The listing builds one solid part. Answer for the finished solid, in the listing's coordinates (mm). A direction names the side the tool comes from. Coordinates: 2 decimals unless noted, no trailing zeros. Order: outer loops, then holes, each group sorted by start corner. A loop starts at its lowest first (then second) coordinate and runs counter-clockwise, first axis right, second up.
from build123d import *

# Parameters (mm, degrees)
SKETCH1_R               = 3.649213309
BOSS_EXTRUDE1_DEPTH     = 2.54
SKETCH1_R_2             = 4.666904756
SKETCH1_R_3             = 2.193652513
BOSS_EXTRUDE1_2_DEPTH   = 2.54
BOSS_EXTRUDE1_3_DEPTH   = 2.54
BOSS_EXTRUDE1_4_DEPTH   = 2.54
SKETCH2_R               = 2.193652513
SKETCH2_R_2             = 2.221197288
SKETCH2_R_3             = 3.649213309
BOSS_EXTRUDE2_DEPTH     = 2.54
SKETCH4_R               = 2.193652513
BOSS_EXTRUDE3_DEPTH     = 2.54
BOSS_EXTRUDE4_REACH     = 60.675
SKETCH5_W               = 19.155946822
SKETCH5_H               = 5.08
SKETCH6_W               = 19.155946822
SKETCH6_H               = 5.30085264
BOSS_EXTRUDE5_DEPTH     = 6.35
SKETCH7_W               = 19.155946822
SKETCH7_H               = 3.58914736
SKETCH7_H_2             = 5.30085264
BOSS_EXTRUDE6_DEPTH     = 6.349999999
CUT_EXTRUDE1_DEPTH      = 113.695579137
BOSS_EXTRUDE7_DEPTH     = 2.54
CUT_EXTRUDE2_DEPTH      = 107.988040918
CUT_EXTRUDE2_DEPTH_BACK = 107.988040918


with BuildPart() as part:
    # Sketch1 → Boss-Extrude1 (new body)
    with BuildSketch(Plane.XY):
        with Locations((-8.202026589, 4.509084108)):
            Circle(SKETCH1_R)
    extrude(amount=BOSS_EXTRUDE1_DEPTH)



with BuildPart() as body_2:
    # Sketch1 → Boss-Extrude1 2 (new body)
    with BuildSketch(Plane.XY):
        with Locations((-3.3, 41.15)):
            Circle(SKETCH1_R_2)
        with Locations((-3.3, 41.15)):
            Circle(SKETCH1_R_3, mode=Mode.SUBTRACT)
    extrude(amount=BOSS_EXTRUDE1_2_DEPTH)


with BuildPart() as body_3:
    # Sketch1 → Boss-Extrude1 3 (new body)
    with BuildSketch(Plane.XY):
        with Locations((-32.26, 41.15)):
            Circle(SKETCH1_R_2)
        with Locations((-32.26, 41.15)):
            Circle(SKETCH1_R_3, mode=Mode.SUBTRACT)
    extrude(amount=BOSS_EXTRUDE1_3_DEPTH)


with BuildPart() as body_4:
    # Sketch1 → Boss-Extrude1 4 (new body)
    with BuildSketch(Plane.XY):
        with Locations((-27.357973411, 4.509084108)):
            Circle(SKETCH1_R)
    extrude(amount=BOSS_EXTRUDE1_4_DEPTH)


with BuildPart() as part_1:
    add(part.part)

    add(body_2.part)  # Boss-Extrude2 merges body 2

    add(body_3.part)  # Boss-Extrude2 merges body 3

    add(body_4.part)  # Boss-Extrude2 merges body 4
    # Sketch2 → Boss-Extrude2 (add)
    # profile 1 of 5: a face of its own
    with BuildSketch(Plane.XY.offset(2.54)):
        with BuildLine():
            ThreePointArc((-8.202026589, 0.859870799), (-10.782410066, 7.089467585), (-4.552813279, 4.509084108))
            Line((-4.552813279, 4.509084108), (1.129473488, 39.680386235))
            ThreePointArc((1.129473488, 39.680386235), (-7.084081624, 38.418566994), (-3.3, 45.816904756))
            Line((-3.3, 45.816904756), (-32.26, 45.816904756))
            ThreePointArc((-32.26, 45.816904756), (-28.96, 44.45), (-27.593095244, 41.15))
            ThreePointArc((-27.593095244, 41.15), (-31.515665024, 36.542835423), (-36.689473488, 39.680386235))
            Line((-36.689473488, 39.680386235), (-31.007186721, 4.509084108))
            ThreePointArc((-31.007186721, 4.509084108), (-27.357973411, 8.158297418), (-23.708760102, 4.509084108))
            ThreePointArc((-23.708760102, 4.509084108), (-24.777589934, 1.928700631), (-27.357973411, 0.859870799))
            Line((-27.357973411, 0.859870799), (-8.202026589, 0.859870799))
        make_face()
    # profile 2 of 5: a face of its own
    with BuildSketch(Plane.XY.offset(2.54)):
        with BuildLine():
            ThreePointArc((-3.3, 45.816904756), (-7.084081624, 38.418566994), (1.129473488, 39.680386235))
            Line((1.129473488, 39.680386235), (1.366904756, 41.15))
            ThreePointArc((1.366904756, 41.15), (0, 44.45), (-3.3, 45.816904756))
        make_face()
        with Locations((-3.3, 41.15)):
            Circle(SKETCH2_R, mode=Mode.SUBTRACT)
    # profile 3 of 5: a face of its own
    with BuildSketch(Plane.XY.offset(2.54)):
        with BuildLine():
            ThreePointArc((-27.593095244, 41.15), (-28.96, 44.45), (-32.26, 45.816904756))
            ThreePointArc((-32.26, 45.816904756), (-35.56, 44.45), (-36.926904756, 41.15))
            Line((-36.926904756, 41.15), (-36.689473488, 39.680386235))
            ThreePointArc((-36.689473488, 39.680386235), (-31.515665024, 36.542835423), (-27.593095244, 41.15))
        make_face()
        with Locations((-32.26, 41.15)):
            Circle(SKETCH2_R_2, mode=Mode.SUBTRACT)
    # profile 4 of 5: a face of its own
    with BuildSketch(Plane.XY.offset(2.54)):
        with Locations(Location((-27.357973411, 4.509084108, 0), (0, 0, 180))):
            Circle(SKETCH2_R_3)
    # profile 5 of 5: a face of its own
    with BuildSketch(Plane.XY.offset(2.54)):
        with Locations((-8.202026589, 4.509084108)):
            Circle(SKETCH2_R_3)
    extrude(amount=BOSS_EXTRUDE2_DEPTH)

    # Sketch4 → Boss-Extrude3 (add)
    with BuildSketch(Plane.XY.offset(5.08)):
        with BuildLine():
            Line((-4.552813279, 4.509084108), (1.366904756, 41.15))
            ThreePointArc((1.366904756, 41.15), (0, 44.45), (-3.3, 45.816904756))
            Line((-3.3, 45.816904756), (-32.26, 45.816904756))
            ThreePointArc((-32.26, 45.816904756), (-35.56, 44.45), (-36.926904756, 41.15))
            Line((-36.926904756, 41.15), (-31.007186721, 4.509084108))
            ThreePointArc((-31.007186721, 4.509084108), (-29.938356889, 1.928700631), (-27.357973411, 0.859870799))
            Line((-27.357973411, 0.859870799), (-8.202026589, 0.859870799))
            ThreePointArc((-8.202026589, 0.859870799), (-5.621643111, 1.928700631), (-4.552813279, 4.509084108))
        make_face()
        with Locations((-3.3, 41.15)):
            Circle(SKETCH4_R, mode=Mode.SUBTRACT)
        with Locations((-32.26, 41.15)):
            Circle(SKETCH4_R, mode=Mode.SUBTRACT)
    extrude(amount=BOSS_EXTRUDE3_DEPTH)

    # Boss-Extrude4: up to this plane
    boss_extrude4_end = Plane(origin=(-92.143596389, -1.511792321, -30.321031804), z_dir=(0, 0.9583363932007225, 0.2856420092826512))
    # Sketch5 → Boss-Extrude4 (add, up to the surface)
    with BuildSketch(Plane.XZ.offset(-0.859870799), mode=Mode.PRIVATE) as boss_extrude4_sk1:
        with Locations((-17.78, 5.08)):
            Rectangle(SKETCH5_W, SKETCH5_H)
    boss_extrude4_tool1 = split(extrude(boss_extrude4_sk1.sketch, amount=BOSS_EXTRUDE4_REACH, mode=Mode.PRIVATE), bisect_by=boss_extrude4_end, keep=Keep.BOTH, mode=Mode.PRIVATE)
    add(boss_extrude4_tool1.solids().sort_by_distance((-17.78, 0.859871, 5.08))[0])

    # Sketch6 → Boss-Extrude5 (add)
    with BuildSketch(Plane(origin=(0, -9.68855673, -2.887773887), x_dir=(1, 0, 0), z_dir=(0, -0.9583363932007226, -0.2856420092826512))):
        with Locations((-17.78, 8.314172293)):
            Rectangle(SKETCH6_W, SKETCH6_H)
    extrude(amount=BOSS_EXTRUDE5_DEPTH)

    # Sketch7 → Boss-Extrude6 (add)
    with BuildSketch(Plane(origin=(0, -15.773992827, -4.701600646), x_dir=(1, 0, 0), z_dir=(0, -0.9583363932007226, -0.2856420092826512))):
        Polygon((-90.857973411, 5.663745973), (-27.357973411, 5.663745973), (-27.357973411, 10.964598613), (-27.357973411, 14.553745973), (-90.857973411, 14.553745973), align=None)
        with Locations((-17.78, 12.759172293)):
            Rectangle(SKETCH7_W, SKETCH7_H)
        with Locations((-17.78, 8.314172293)):
            Rectangle(SKETCH7_W, SKETCH7_H_2)
        Polygon((-8.202026589, 10.964598613), (-8.202026589, 5.663745973), (55.297973411, 5.663745973), (55.297973411, 14.553745973), (-8.202026589, 14.553745973), align=None)
    extrude(amount=-BOSS_EXTRUDE6_DEPTH)

    # Sketch9 → Cut-Extrude1 (cut, through all)
    with BuildSketch(Plane(origin=(0, 45.816904756, 0), x_dir=(1, 0, 0), z_dir=(0, 1, 0))):
        Polygon((-3.3, -7.62), (-17.78, -7.62), (-17.78, -45.955901378), (77.021856541, -45.955901378), (77.021856541, -7.62), align=None)
        Polygon((-17.78, -45.955901378), (-17.78, -7.62), (-32.26, -7.62), (-120.520571542, -7.62), (-120.520571542, -45.955901378), align=None)
    extrude(amount=-CUT_EXTRUDE1_DEPTH, mode=Mode.SUBTRACT)

    # Sketch10 → Boss-Extrude7 (add)
    with BuildSketch(Plane(origin=(0, -1.61780378, 5.427773887), x_dir=(-1, 0, 0), z_dir=(0, 0.28564200928265115, -0.9583363932007226))):
        Polygon((27.357973411, -10.109766049), (8.202026589, -10.109766049), (-55.297973411, -10.109766049), (-55.297973411, -16.459766048), (90.857973411, -16.459766048), (90.857973411, -10.109766049), align=None)
    extrude(amount=BOSS_EXTRUDE7_DEPTH)

    # Sketch11 → Cut-Extrude2 (cut, two sides: drawn at the far end of the back side and taken through both)
    with BuildSketch(Plane(origin=(0, -9.688556731, -2.887773887), x_dir=(1, 0, 0), z_dir=(0, 0.9583363932007284, 0.28564200928263184)).offset(-CUT_EXTRUDE2_DEPTH_BACK)):
        with BuildLine():
            Line((-41.109605197, -5.294172293), (-83.237973411, -5.294172293))
            ThreePointArc((-83.237973411, -5.294172293), (-84.475410278, -5.806735425), (-84.987973411, -7.044172293))
            ThreePointArc((-84.987973411, -7.044172293), (-84.475410278, -8.28160916), (-83.237973411, -8.794172293))
            Line((-83.237973411, -8.794172293), (-41.109605197, -8.794172293))
            ThreePointArc((-41.109605197, -8.794172293), (-39.359605197, -7.044172293), (-41.109605197, -5.294172293))
        make_face()
        with BuildLine():
            Line((5.549605197, -8.794172293), (47.677973411, -8.794172293))
            ThreePointArc((47.677973411, -8.794172293), (49.427973411, -7.044172293), (47.677973411, -5.294172293))
            Line((47.677973411, -5.294172293), (5.549605197, -5.294172293))
            ThreePointArc((5.549605197, -5.294172293), (3.799605197, -7.044172293), (5.549605197, -8.794172293))
        make_face()
    extrude(amount=CUT_EXTRUDE2_DEPTH + CUT_EXTRUDE2_DEPTH_BACK, mode=Mode.SUBTRACT)


solid = part_1.part
(1) The mould has two halves that part along X. Classify faces 6 (the flat face through (-27, 5, 0)), 7 (the flat face through (-8.202, -5, 5)), 8 (the flat face through (26.909, -14.286, 1.266)): pulls with the +X half, pulls with the -X half, needs draft (parallel to the pull), parting line crosses it, or undercut.
(2) Find the intervals of material crossed by probe 1 along Y at (x, z) = (-32.26, 1.55); probe 2 along Z at (x, y) = (-14, 43); probe 3 along Y at (x, z) = (-37, 6), in increasing order.
(3) Find section B-B on y = 16. Determine the outline of the cut face in (x, z).
(4) Find section C-C on x = -26. Determine the outline of the cut face in (y, z), then the cut area to 3 significant figures.
(5) Given pin 1 Ø2 at (x, z) = (-73, -0.5) entering from +Y; pin 2 Ø7.5 at (x, y) = (-3.5, 42.5) entering from -Z; pin 3 Ø2.5 at (x, y) = (-32.26, 41.15) entering from +Z; pin 4 Ø4 at (x, z) = (0.5, 0.5) entering from +Y, each flat-ended and moving along its own axis, determine where each tip first touches the part or whether it passes through.
(6) Find section D-D on x = -10. Determine the outline of the cut face in (y, z).
(7) A tool of negligible diameter and unlimited length cuts with its end or side. For faces 1 (the cylindrical face through (-35.7, 44.304, 2.91)), 2 (the cylindrical face through (49.428, -14.797, 2.98)), 3 (the flat face through (-62.47, -15.29, 4.62)), 4 (the flat face through (-1, 40, 0)), 5 (the flat face through (-61.879, -14.286, 1.266)), from which of +Z, -Z, +X, -X, +Y, -Y can it reach the whole face along a straight path? Write none if from no direction.
(8) Find section A-A on x = -73. Determine the outline of the cut face in (y, z), then the cut area to 3 significant figures.
Resolved:
1. face 6: needs draft
1. face 7: pulls with the +X half
1. face 8: undercut
2. probe 1: y = -17.64 to -11.01, 36.48 to 38.96, 43.34 to 45.82
2. probe 2: z = 2.54 to 7.62
2. probe 3: y = -18.96 to -12.34
3. outline: (-32.86, 2.54) - (-2.7, 2.54) - (-2.7, 7.62) - (-32.86, 7.62) - close
4. outline: (-19.45, 7.62) - (-16.67, -1.71) - (-10.58, 0.11) - (-11.31, 2.54) - (1.12, 2.54) - (1.12, 0) - (7.9, 0) - (7.9, 2.54) - (45.82, 2.54) - (45.82, 7.62) - close
4. area: 367 mm2
5. pin 1: stops at y = -10.58
5. pin 2: stops at z = 0
5. pin 3: passes through
5. pin 4: stops at y = 45.46
6. outline: (-19.45, 7.62) - (-16.67, -1.71) - (-10.58, 0.11) - (-11.31, 2.54) - (1.33, 2.54) - (1.33, 0) - (7.68, 0) - (7.68, 2.54) - (45.82, 2.54) - (45.82, 7.62) - close
7. face 1: -Z
7. face 2: none
7. face 3: +Y
7. face 4: -Z, +X, -X, +Y
7. face 5: -Y
8. outline: (-19.45, 7.62) - (-18.29, 3.73) - (-12.2, 5.54) - (-12.82, 7.62) - close; (-17.29, 0.37) - (-16.67, -1.71) - (-10.58, 0.11) - (-11.2, 2.19) - close
8. area: 33.6 mm2
